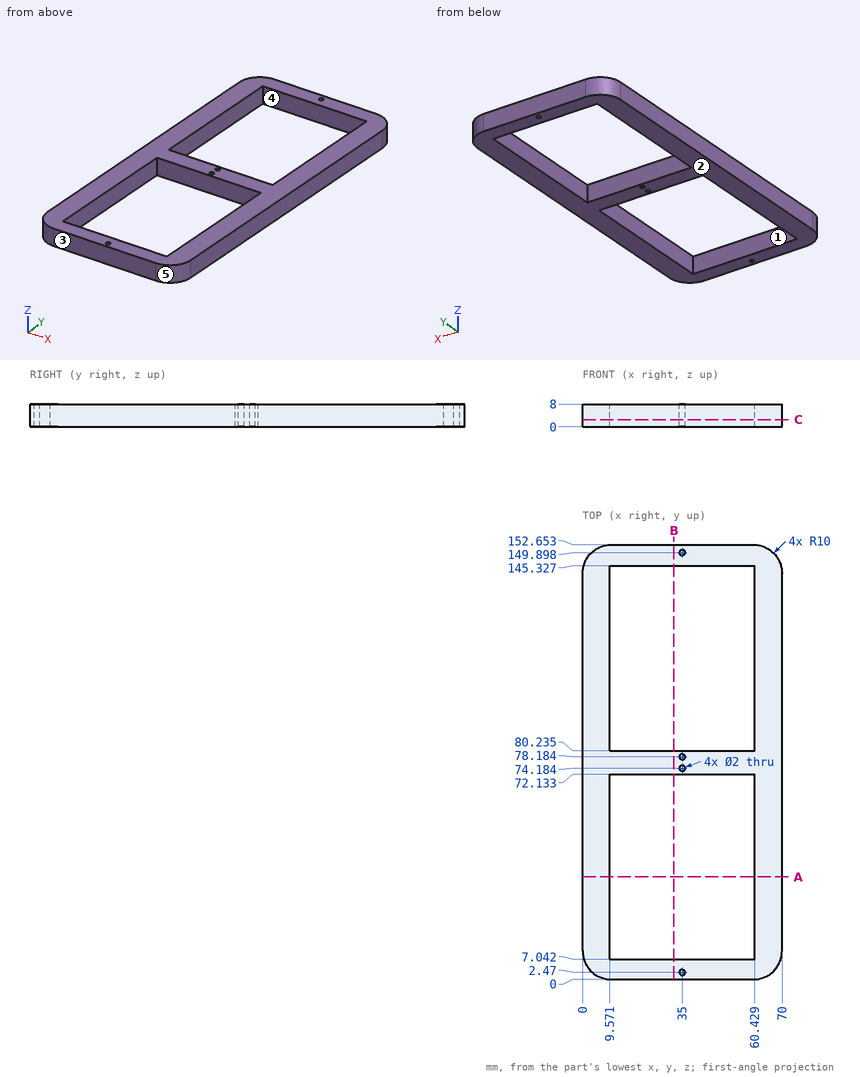
Can you work these out from the drawing? Everything is in mm from the part's minimum corner. A direction names the side the tool comes from. Round coordinates to 2 decimals unless told otherwise and drop trailing zeros. Loops run counter-clockwise (first coordinate to the right, second up) from the corner with the lowest first, then second, coordinate; pieces in that order, holes last. Notation, with made-up numbers: (70.5, 83) -> (122.5, 83) arc R30 ccw to (122.5, 121) -> close; hole circle Ø1 at (-34, 20). An arc over 180 degrees is marked (long way). Answer in a Markdown table with one row per item.
Item 1: Suppose I cut it at C-C, the plane z = 2.5. List the corners of the cut face in (x, y) for me (1 decimal), plus the area to 3 significant figures.
Answer block:
| item | result |
|---|---|
| outline | (0, 10) arc R10 ccw to (10, 0) -> (60, 0) arc R10 ccw to (70, 10) -> (70, 142.7) arc R10 ccw to (60, 152.7) -> (10, 152.7) arc R10 ccw to (0, 142.7) -> close; hole (9.6, 7) -> (60.4, 7) -> (60.4, 72.1) -> (9.6, 72.1) -> close; hole (9.6, 80.2) -> (60.4, 80.2) -> (60.4, 145.3) -> (9.6, 145.3) -> close; hole circle Ø2 at (35, 2.5); hole circle Ø2 at (35, 74.2); hole circle Ø2 at (35, 78.2); hole circle Ø2 at (35, 149.9) |
| area | 3,970 mm² |
Item 2: On a 3-axis mill with a long thin cutter (end or side, diameter ignored), from which of +Z, -Z, +X, -X, +Y, -Y can I reach the whole of each face in a straight line? I mean the marked faces 1 and 2. Say none if no direction works.
Answer block:
| item | result |
|---|---|
| face 1 | +Z, -Z |
| face 2 | -Z, +X, -X, +Y, -Y |
Item 3: Suppose I cut it at A-A, the plane y = 36. List the corners of the cut face in (x, z) for me, plus the area to 3 significant figures.
Answer block:
| item | result |
|---|---|
| outline | (0, 0) -> (9.57, 0) -> (9.57, 8) -> (0, 8) -> close; (60.43, 0) -> (70, 0) -> (70, 8) -> (60.43, 8) -> close |
| area | 153 mm² |
Item 4: Will this pin go through, and if not, where does the flat tip stop? P1, Ø1.2, axis at x = 35, y = 2.47, coming from the +Z side.
Answer block:
| item | result |
|---|---|
| P1 | through |
Item 5: We'd pull the mould along X, two halves only. Please class the marked faces 3, 4 and 5: released by +X, released by -X, zero draft, split by the parting line, or undercut.
Answer block:
| item | result |
|---|---|
| face 3 | zero draft |
| face 4 | undercut |
| face 5 | released by +X |
Item 6: Suppose I cut it at B-B, the plane x = 32. List the corners of the cut face in (y, z) for me (1 decimal).
Answer block:
| item | result |
|---|---|
| outline | (0, 0) -> (7, 0) -> (7, 8) -> (0, 8) -> close; (72.1, 0) -> (80.2, 0) -> (80.2, 8) -> (72.1, 8) -> close; (145.3, 0) -> (152.7, 0) -> (152.7, 8) -> (145.3, 8) -> close |
Item 7: If I drill on probe 1 along Y at (x, z) = (11, 5.75) (1 decimal); probe 2 along X at (y, z) = (54, 1.5); probe 3 along Y at (x, z) = (9.5, 4.25), over which ranges is the centre line in solid material (lowest first)?
Answer block:
| item | result |
|---|---|
| probe 1 | 0 to 7, 72.1 to 80.2, 145.3 to 152.7 |
| probe 2 | 0 to 9.57, 60.43 to 70 |
| probe 3 | 0.01 to 152.64 |
